from build123d import *

# Parameters (mm, degrees)
ESBO_O1_R                  = 46.55
RESSALTO_EXTRUS_O1_DEPTH   = 49
CORTE_EXTRUS_O2_DEPTH      = 83.0658577
CORTE_EXTRUS_O2_DEPTH_BACK = 83.0658577
CORTE_EXTRUS_O10_START     = -49
ESBO_O3_OUTSIDE_W          = 79.756
ESBO_O3_OUTSIDE_H          = 123.856
ESBO_O3_OUTSIDE_R          = 9
CORTE_EXTRUS_O10_DEPTH     = 26
CORTE_EXTRUS_O11_START     = 49
ESBO_O6_OUTSIDE_W          = 79.756
ESBO_O6_OUTSIDE_H          = 123.856
ESBO_O6_OUTSIDE_R          = 9
CORTE_EXTRUS_O11_DEPTH     = 26
ESBO_O7_OUTSIDE_W          = 79.756
ESBO_O7_OUTSIDE_H          = 123.856
ESBO_O7_OUTSIDE_R          = 5.5
CORTE_EXTRUS_O12_DEPTH     = 10.5
ESBO_O8_OUTSIDE_W          = 79.756
ESBO_O8_OUTSIDE_H          = 123.856
ESBO_O8_OUTSIDE_R          = 5.5
CORTE_EXTRUS_O13_DEPTH     = 10.5
ESBO_O9_W                  = 16
ESBO_O9_H                  = 36.861601527


with BuildPart() as part:
    # Esboço1 → Ressalto-extrusão1 (new, symmetric)
    with BuildSketch(Plane(origin=(0, 0, 0), x_dir=(0, 0, -1), z_dir=(1, 0, 0))):
        Circle(ESBO_O1_R)
    extrude(amount=RESSALTO_EXTRUS_O1_DEPTH, both=True)

    # Esboço2 → Corte-extrusão2 (cut, two sides: drawn at the far end of the back side and taken through both)
    with BuildSketch(Plane(origin=(0, 0, 0), x_dir=(0, 0, -1), z_dir=(1, 0, 0)).offset(-CORTE_EXTRUS_O2_DEPTH_BACK)):
        with BuildLine():
            Line((-24.5, -20.172926622), (-24.5, 39.580961332))
            ThreePointArc((-24.5, 39.580961332), (-46.55, 0), (-24.5, -39.580961332))
            Line((-24.5, -39.580961332), (-24.5, -20.172926622))
        make_face()
        with BuildLine():
            ThreePointArc((-24.5, -39.580961332), (-12.735948139, -44.773855374), (0, -46.55))
            Line((0, -46.55), (-24.5, -20.172926622))
            Line((-24.5, -20.172926622), (-24.5, -39.580961332))
        make_face()
        with BuildLine():
            ThreePointArc((46.55, 0), (40.665572048, 22.654221461), (24.5, 39.580961332))
            Line((24.5, 39.580961332), (24.5, 20.172926622))
            Line((24.5, 20.172926622), (24.5, -39.580961332))
            ThreePointArc((24.5, -39.580961332), (40.665572048, -22.654221461), (46.55, 0))
        make_face()
        with BuildLine():
            Line((24.5, 20.172926622), (24.5, 39.580961332))
            ThreePointArc((24.5, 39.580961332), (12.735948139, 44.773855374), (0, 46.55))
            Line((0, 46.55), (24.5, 20.172926622))
        make_face()
    extrude(amount=CORTE_EXTRUS_O2_DEPTH + CORTE_EXTRUS_O2_DEPTH_BACK, mode=Mode.SUBTRACT)

    # Esboço3 outside → Corte-extrusão10 (cut)
    with BuildSketch(Plane(origin=(0, 0, 0), x_dir=(0, 0, -1), z_dir=(1, 0, 0)).offset(CORTE_EXTRUS_O10_START)):
        Rectangle(ESBO_O3_OUTSIDE_W, ESBO_O3_OUTSIDE_H)
        with Locations(Location((0, 0, 0), (0, 0, 180))):
            Circle(ESBO_O3_OUTSIDE_R, mode=Mode.SUBTRACT)
    extrude(amount=CORTE_EXTRUS_O10_DEPTH, mode=Mode.SUBTRACT)

    # Esboço6 outside → Corte-extrusão11 (cut)
    with BuildSketch(Plane(origin=(0, 0, 0), x_dir=(0, 0, -1), z_dir=(1, 0, 0)).offset(CORTE_EXTRUS_O11_START)):
        Rectangle(ESBO_O6_OUTSIDE_W, ESBO_O6_OUTSIDE_H)
        with Locations(Location((0, 0, 0), (0, 0, 180))):
            Circle(ESBO_O6_OUTSIDE_R, mode=Mode.SUBTRACT)
    extrude(amount=-CORTE_EXTRUS_O11_DEPTH, mode=Mode.SUBTRACT)

    # Esboço7 outside → Corte-extrusão12 (cut)
    with BuildSketch(Plane(origin=(49, 0, 0), x_dir=(0, 0, -1), z_dir=(1, 0, 0))):
        Rectangle(ESBO_O7_OUTSIDE_W, ESBO_O7_OUTSIDE_H)
        Circle(ESBO_O7_OUTSIDE_R, mode=Mode.SUBTRACT)
    extrude(amount=-CORTE_EXTRUS_O12_DEPTH, mode=Mode.SUBTRACT)

    # Esboço8 outside → Corte-extrusão13 (cut)
    with BuildSketch(Plane.ZY.offset(49)):
        Rectangle(ESBO_O8_OUTSIDE_W, ESBO_O8_OUTSIDE_H)
        with Locations(Location((0, 0, 0), (0, 0, 180))):
            Circle(ESBO_O8_OUTSIDE_R, mode=Mode.SUBTRACT)
    extrude(amount=-CORTE_EXTRUS_O13_DEPTH, mode=Mode.SUBTRACT)

    # Esboço9 → Corte-Revolução1 (revolve, cut)
    with BuildSketch(Plane.XY, mode=Mode.PRIVATE) as corte_revolu_o1_sk:
        with Locations((0, 32.980800763)):
            Rectangle(ESBO_O9_W, ESBO_O9_H)
    revolve(corte_revolu_o1_sk.sketch.rotate(Axis((-1000, 0, 0), (1, 0, 0)), 90), axis=Axis((-1000, 0, 0), (1, 0, 0)), mode=Mode.SUBTRACT)


solid = part.part
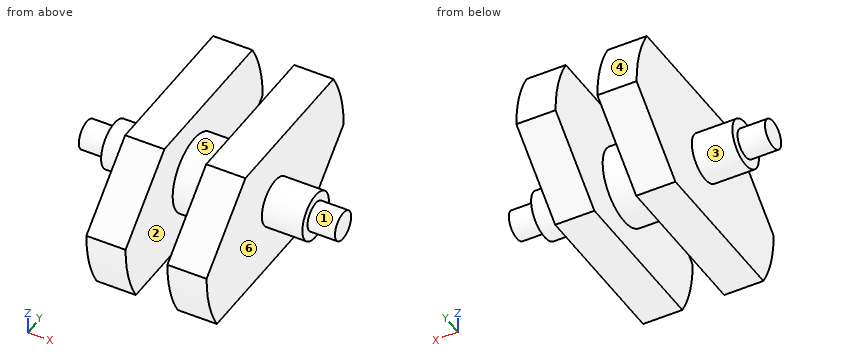
Can you work these out from the model? Positions are in its coordinate system, mm. Face numbers are marked on the shaded views. A direction names the side the tool comes from. Round coordinates to 2 decimals unless told otherwise and drop trailing zeros. Loops run counter-clockwise (first coordinate to the right, second up) from the corner with the lowest first, then second, coordinate; pieces in that order, holes last. Notation, with made-up numbers: (25, -17) - (56, -17) arc R22 ccw to (56, 9) - close; hole circle Ø3 at (-31, 30). An arc over 180 degrees is marked (long way). Answer in a Markdown table with one row per item. Add a question column.
Q1. I need wall thicknesses on L1, parallel to X at y = -22, z = -2; L2, parallel to X at y = 2.5, z = -8; L3, parallel to Y at x = -5, z = -9.5. Which ranges of each line are inside material? Lowest first, please.
Q2. Which directions (+Z, -Z, +X, -X, +Y, -Y) give clear straight access to the entire face, cutting with the end or side of a thin tool? Please do the marked faces 1, 2 and 3.
Q3. For pin 1 Ø10 at (y, z) = (-31, 0.5) entering from +X; pin 2 Ø12 at (x, z) = (-1, 4) entering from +Y; pin 3 Ø5 at (x, z) = (22.5, -12.5) entering from +Y, each with a flat end and sliding along its axis, tell me the tip position at first contact or that it passes through.
Q4. I want a section at C-C on x = 16. List the corners of the cut face in (y, z) for me, and give its area (3 significant figures).
Q5. We'd pull the mould along X, two halves only. Please class the marked faces 4, 5 and 6: pulls with the +X half, pulls with the -X half, needs draft (parallel to the pull), parting line crosses it, or undercut.
Q6. I want a section at D-D on x = -33.5. List the corners of the cut face in (y, z) for me.
Q7. I want a section at B-B on y = 0. List the corners of the cut face in (x, z) for me.
Q8. I want a section at A-A on y = 32. List the corners of the cut face in (x, z) for me, and give its area (3 significant figures).
A:
| question | item | result |
|---|---|---|
| 1 | L1 | -23 to -8, 8 to 23 |
| 1 | L2 | -38.5 to 38.5 |
| 1 | L3 | -11.02 to 11.02 |
| 2 | face 1 | +X |
| 2 | face 2 | none |
| 2 | face 3 | -X |
| 3 | pin 1 | x = 23 |
| 3 | pin 2 | y = 14.55 |
| 3 | pin 3 | y = 35.78 |
| 4 | outline | (-46.55, 0) arc R46.55 ccw to (-39.58, -24.5) - (20.17, -24.5) - (46.55, 0) arc R46.55 ccw to (39.58, 24.5) - (-20.17, 24.5) - close |
| 4 | area | 3,810 mm^2 |
| 5 | face 4 | needs draft |
| 5 | face 5 | undercut |
| 5 | face 6 | pulls with the +X half |
| 6 | outline | circle Ø18 at (0, 0) |
| 7 | outline | (-49, -5.5) - (-38.5, -5.5) - (-38.5, -9) - (-23, -9) - (-23, -24.5) - (-8, -24.5) - (-8, -14.55) - (8, -14.55) - (8, -24.5) - (23, -24.5) - (23, -9) - (38.5, -9) - (38.5, -5.5) - (49, -5.5) - (49, 5.5) - (38.5, 5.5) - (38.5, 9) - (23, 9) - (23, 24.5) - (8, 24.5) - (8, 14.55) - (-8, 14.55) - (-8, 24.5) - (-23, 24.5) - (-23, 9) - (-38.5, 9) - (-38.5, 5.5) - (-49, 5.5) - close |
| 8 | outline | (-23, -13.51) - (-8, -13.51) - (-8, 24.5) - (-23, 24.5) - close; (8, -13.51) - (23, -13.51) - (23, 24.5) - (8, 24.5) - close |
| 8 | area | 1,140 mm^2 |
